Part model, mm, in its own coordinate system. A direction names the side the tool comes from. Round coordinates to 2 decimals unless told otherwise and drop trailing zeros.
from build123d import *

# Parameters (mm, degrees)
F0_W      = 635.6985
F0_H      = 38.1
F0_W_2    = 674.878
F1_DEPTH  = 19.05
F2_W      = 657.2885064902
F2_H      = 254
F2_W_2    = 553.1485062082
F2_H_2    = 160.0199994359
F3_DEPTH  = 19.05
F2_W_3    = 560.7685060475
F2_H_3    = 165.0999991145
F4_DEPTH  = 19.05
F2_H_4    = 234.95
F2_W_4    = 542.9885064902
F2_H_5    = 120.65
F5_DEPTH  = 19.05
F6_DEPTH  = 6.35
F2_W_5    = 700.278
F2_W_6    = 585.978
F7_DEPTH  = 19.05
F8_DEPTH  = 6.35
F9_DEPTH  = 6.35
F2_W_7    = 335.8515
F2_H_6    = 495.3
F2_W_8    = 234.2515
F2_H_7    = 406.4
F10_DEPTH = 19.05
F11_DEPTH = 6.35
F2_W_9    = 661.0985
F2_W_10   = 546.7985
F2_H_8    = 139.7
F12_DEPTH = 19.05
F13_DEPTH = 12.7
F14_DEPTH = 6.35
F15_DEPTH = 6.35
F16_DEPTH = 6.35


with BuildPart() as f1:
    # F0 (on Front) → F1 (new body)
    with BuildSketch(Plane.XZ):
        Polygon((-986.4497834325, 548.455909781), (-1024.5497834325, 548.455909781), (-1024.5497834325, -270.694090219), (-986.4497834325, -270.694090219), (-986.4497834325, -232.594090219), (-986.4497834325, -3.994090219), (-986.4497834325, 34.105909781), (-986.4497834325, 262.705909781), (-986.4497834325, 300.805909781), (-986.4497834325, 510.355909781), align=None)
        with Locations((-668.6005334325, -251.644090219)):
            Rectangle(F0_W, F0_H)
        with Locations((-668.6005334325, 15.055909781)):
            Rectangle(F0_W, F0_H)
        with Locations((-668.6005334325, 281.755909781)):
            Rectangle(F0_W, F0_H)
        with Locations((-668.6005334325, 529.405909781)):
            Rectangle(F0_W, F0_H)
        Polygon((-312.6512834325, 548.455909781), (-350.7512834325, 548.455909781), (-350.7512834325, 510.355909781), (-350.7512834325, 300.805909781), (-350.7512834325, 262.705909781), (-350.7512834325, 34.105909781), (-350.7512834325, -3.994090219), (-350.7512834325, -232.594090219), (-350.7512834325, -270.694090219), (-312.6512834325, -270.694090219), (-312.6512834325, -232.594090219), (-312.6512834325, 262.705909781), (-312.6512834325, 300.805909781), (-312.6512834325, 510.355909781), align=None)
        with Locations((24.7877165675, 529.405909781)):
            Rectangle(F0_W_2, F0_H)
        with Locations((24.7877165675, 281.755909781)):
            Rectangle(F0_W_2, F0_H)
        with Locations((24.7877165675, -251.644090219)):
            Rectangle(F0_W_2, F0_H)
        Polygon((400.3267165675, 548.455909781), (362.2267165675, 548.455909781), (362.2267165675, 510.355909781), (362.2267165675, 300.805909781), (362.2267165675, 262.705909781), (362.2267165675, -232.594090219), (362.2267165675, -270.694090219), (400.3267165675, -270.694090219), (400.3267165675, -232.594090219), (400.3267165675, -3.994090219), (400.3267165675, 34.105909781), (400.3267165675, 262.705909781), (400.3267165675, 300.805909781), (400.3267165675, 510.355909781), align=None)
        with Locations((718.1759665675, 15.055909781)):
            Rectangle(F0_W, F0_H)
        with Locations((718.1759665675, 281.755909781)):
            Rectangle(F0_W, F0_H)
        with Locations((718.1759665675, 529.405909781)):
            Rectangle(F0_W, F0_H)
        with Locations((718.1759665675, -251.644090219)):
            Rectangle(F0_W, F0_H)
        Polygon((1036.0252165675, -270.694090219), (1074.1252165675, -270.694090219), (1074.1252165675, 548.455909781), (1036.0252165675, 548.455909781), (1036.0252165675, 510.355909781), (1036.0252165675, 300.805909781), (1036.0252165675, 262.705909781), (1036.0252165675, 34.105909781), (1036.0252165675, -3.994090219), (1036.0252165675, -232.594090219), align=None)
    extrude(amount=-F1_DEPTH)

    # F2 (on face) → F3 (join)
    with BuildSketch(Plane.XZ):
        with Locations((-670.5055301874, -118.294090219)):
            Rectangle(F2_W, F2_H)
        with Locations((-675.5855300463, -118.294090219)):
            Rectangle(F2_W_2, F2_H_2, mode=Mode.SUBTRACT)
    extrude(amount=F3_DEPTH)

    # F2 (on face) → F4 (join)
    with BuildSketch(Plane.XZ):
        with Locations((-670.5055301874, 148.405909781)):
            Rectangle(F2_W, F2_H)
        with Locations((-674.315529966, 148.405909781)):
            Rectangle(F2_W_3, F2_H_3, mode=Mode.SUBTRACT)
    extrude(amount=F4_DEPTH)

    # F2 (on face) → F5 (join)
    with BuildSketch(Plane.XZ):
        with Locations((-670.5055301874, 405.580909781)):
            Rectangle(F2_W, F2_H_4)
        with Locations((-670.5055301874, 405.580909781)):
            Rectangle(F2_W_4, F2_H_5, mode=Mode.SUBTRACT)
    extrude(amount=F5_DEPTH)

    # F2 (on face) → F6 (join)
    with BuildSketch(Plane.XZ):
        with Locations((-670.5055301874, 405.580909781)):
            Rectangle(F2_W_4, F2_H_5)
    extrude(amount=F6_DEPTH)

    # F2 (on face) → F7 (join)
    with BuildSketch(Plane.XZ):
        with Locations((24.7877165675, 405.580909781)):
            Rectangle(F2_W_5, F2_H_4)
        with Locations((24.7877165675, 405.580909781)):
            Rectangle(F2_W_6, F2_H_5, mode=Mode.SUBTRACT)
    extrude(amount=F7_DEPTH)

    # F2 (on face) → F8 (join)
    with BuildSketch(Plane.XZ):
        with Locations((24.7877165675, 405.580909781)):
            Rectangle(F2_W_6, F2_H_5)
    extrude(amount=F8_DEPTH)

    # F2 (on face) → F9 (join)
    with BuildSketch(Plane.XZ):
        with Locations((-674.315529966, 148.405909781)):
            Rectangle(F2_W_3, F2_H_3)
        with Locations((-675.5855300463, -118.294090219)):
            Rectangle(F2_W_2, F2_H_2)
    extrude(amount=F9_DEPTH)

    # F2 (on face) → F10 (join)
    with BuildSketch(Plane.XZ):
        Polygon((23.2002165675, 275.405909781), (-325.3512834325, 275.405909781), (-325.3512834325, -245.294090219), (23.2002165675, -245.294090219), (23.2002165675, -232.594090219), (-312.6512834325, -232.594090219), (-312.6512834325, 262.705909781), (23.2002165675, 262.705909781), align=None)
        with Locations((-144.7255334325, 15.055909781)):
            Rectangle(F2_W_7, F2_H_6)
        with Locations((-151.0755334325, 15.055909781)):
            Rectangle(F2_W_8, F2_H_7, mode=Mode.SUBTRACT)
        Polygon((26.3752165675, 275.405909781), (26.3752165675, 262.705909781), (362.2267165675, 262.705909781), (362.2267165675, -232.594090219), (26.3752165675, -232.594090219), (26.3752165675, -245.294090219), (374.9267165675, -245.294090219), (374.9267165675, 275.405909781), align=None)
        with Locations((194.3009665675, 15.055909781)):
            Rectangle(F2_W_7, F2_H_6)
        with Locations((200.6509665675, 15.055909781)):
            Rectangle(F2_W_8, F2_H_7, mode=Mode.SUBTRACT)
    extrude(amount=F10_DEPTH)

    # F2 (on face) → F11 (join)
    with BuildSketch(Plane.XZ):
        with Locations((-151.0755334325, 15.055909781)):
            Rectangle(F2_W_8, F2_H_7)
        with Locations((200.6509665675, 15.055909781)):
            Rectangle(F2_W_8, F2_H_7)
    extrude(amount=F11_DEPTH)

    # F2 (on face) → F12 (join)
    with BuildSketch(Plane.XZ):
        with Locations((718.1759665675, 405.580909781)):
            Rectangle(F2_W_9, F2_H_4)
        with Locations((718.1759665675, 405.580909781)):
            Rectangle(F2_W_10, F2_H_5, mode=Mode.SUBTRACT)
        with Locations((718.1759665675, 148.405909781)):
            Rectangle(F2_W_9, F2_H)
        with Locations((718.1759665675, 148.405909781)):
            Rectangle(F2_W_10, F2_H_8, mode=Mode.SUBTRACT)
        with Locations((718.1759665675, -118.294090219)):
            Rectangle(F2_W_9, F2_H)
        with Locations((718.1759665675, -118.294090219)):
            Rectangle(F2_W_10, F2_H_8, mode=Mode.SUBTRACT)
    extrude(amount=F12_DEPTH)

    # F2 (on face) → F13 (join)
    with BuildSketch(Plane.XZ):
        with Locations((718.1759665675, 405.580909781)):
            Rectangle(F2_W_10, F2_H_5)
    extrude(amount=F13_DEPTH)

    # F14 (cut): a face of the model
    f14_faces = [f1.faces().sort_by_distance(p)[0] for p in [
        (718.1759665675, -12.7, 405.580909781),
    ]]
    extrude(f14_faces, amount=F14_DEPTH, mode=Mode.SUBTRACT)

    # F2 (on face) → F15 (cut)
    with BuildSketch(Plane.XZ):
        with Locations((718.1759665675, 405.580909781)):
            Rectangle(F2_W_10, F2_H_5)
    extrude(amount=-F15_DEPTH, mode=Mode.SUBTRACT)

    # F2 (on face) → F16 (join)
    with BuildSketch(Plane.XZ):
        with Locations((718.1759665675, 148.405909781)):
            Rectangle(F2_W_10, F2_H_8)
        with Locations((718.1759665675, -118.294090219)):
            Rectangle(F2_W_10, F2_H_8)
    extrude(amount=F16_DEPTH)


solid = f1.part
Q1. Tool access for faces 3 (the flat face through (-679, -6.35, -117)), 4 (the flat face through (-270, -19.05, 19)), 5 (the flat face through (-147, 0, 19)): list every direction of +Z, -Z, +X, -X, +Y, -Y with a clear straight run to the whole face (end or side of a thin tool).
Q2. Saw through at A-A, the plane y = 7.5. Give the number of separate pieces and of enclosed holes in the cut face, and give its area (3 significant figures).
Q3. Drop flat-ended pins along their axis: P1, Ø6, axis at y = -13, z = 247, coming from the +X side; P2, Ø2, axis at x = -801, y = -10.5, coming from the -Z side; P3, Ø9.5, axis at y = -13.5, z = -75, coming from the -X side. Give the stop position or say it passes through.
Q4. Wall check: line 1 (X direction, y = 5, z = -31.5); line 2 (Z direction, x = -893, y = -2.5); line 3 (Z direction, x = -720, y = 2.5). Give the ranges that are in metal, low to high.
Q5. Two-plate mould, pull along X, no slides. Class faces 1 (the flat face through (714, -19.05, 235)), 2 (the flat face through (714, -12.7, 406)): released by +X, released by -X, zero draft, split by the parting line, or undercut.
Computed:
1. face 3: -Y
1. face 4: +Z, -Z, +X, -X, -Y
1. face 5: +Y
2. separate pieces: 1
2. enclosed holes: 8
2. area: 396,000 mm2
3. P1: stops at x = 1048.73
3. P2: stops at z = -245.29
3. P3: stops at x = -999.15
4. line 1: x = -1024.55 to -986.45, -350.75 to -312.65, 362.23 to 400.33, 1036.03 to 1074.13
4. line 2: z = -245.29 to 8.71, 21.41 to 275.41, 288.11 to 523.06
4. line 3: z = -270.69 to -232.59, -3.99 to 34.11, 262.71 to 300.81, 510.36 to 548.46
5. face 1: zero draft
5. face 2: undercut
